Check sheet for the modelled part. Datum: model origin and axes. Units: mm. Face numbers are marked on the shaded views. A direction names the side the tool comes from. Round coordinates to 2 decimals unless told otherwise and drop trailing zeros. Order: outer loops, then holes, each group sorted by start corner. A loop starts at its lowest first (then second) coordinate and runs counter-clockwise, first axis right, second up.
```python
from build123d import *

# Parameters (mm, degrees)
F2_R    = 2.99999
F3_SIZE = 2


# Not quite as in the source:
# - a fillet or chamfer is up to 0.001 mm smaller than in the source, because OpenCascade refuses the exact size


with BuildPart() as f1:
    # F0 (on Top) → F1 (revolve)
    with BuildSketch(Plane.XY):
        Polygon((-62.0045285772, 2), (-62.0045285772, -10), (45.9954714228, -10), (45.9954714228, -5), (36.4192584626, 0), (31.4192584626, 0), (31.4192584626, -3), (26.4192584626, -3), (26.4192584626, 0), (21.4192584626, 0), (21.4192584626, 8), (11.4192584626, 8), (11.4192584626, 11), (1.4192584626, 11), (1.4192584626, 8), (-18.5807415374, 8), (-18.5807415374, 2), align=None)
    revolve(axis=Axis((-8.0045285772, -10, 0), (1, 0, 0)))

    # F2 (radius 3 in the source; OpenCascade refuses exactly that, so slightly less here)
    f2_edges = [f1.edges().sort_by_distance(p)[0] for p in [
        (-18.580742, -28, 0),
        (-18.580742, -22, 0),
    ]]
    fillet(f2_edges, radius=F2_R)

    # F3
    f3_edges = [f1.edges().sort_by_distance(p)[0] for p in [
        (21.419258, -28, 0),
        (-62.004529, -22, 0),
    ]]
    chamfer(f3_edges, length=F3_SIZE)


solid = f1.part
```
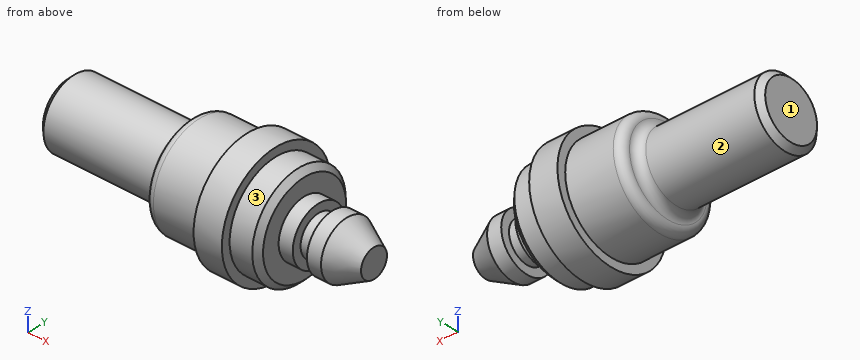
Item 1: Sectioned sample at A-A (x = -24). Record the cut outline in (y, z), and give its area (3 significant figures).
Answer:
outline: circle Ø24 at (-10, 0)
area: 452 mm2
Item 2: Sectioned sample at B-B (x = 32.5). Record the cut outline in (y, z).
Answer:
outline: circle Ø20 at (-10, 0)
Item 3: Scan lines: line 1 along X through (y, z) = (-10, -18.5); line 2 along Z through (x, y) = (10, -2); line 3 along X through (y, z) = (-7.5, -10). Record each from-to range of solid material in increasing order.
Answer:
line 1: x = 1.42 to 11.42
line 2: z = -19.42 to 19.42
line 3: x = -61.7 to 21.42
Item 4: Go/stop test with flat-tipped pins: P1, Ø1, axis at x = 23.5, z = 13.5, coming from the -Y side; P2, Ø12, axis at x = -4, z = -6.5, coming from the +Y side; P3, Ø5, axis at x = -32.5, y = -7, coming from the -Z side; P4, Ø2, axis at y = -24, z = -6.5, coming from the +X side. Record where each tip stops, or that it passes through.
Answer:
P1: passes through
P2: stops at y = 10.63
P3: stops at z = -11.99
P4: stops at x = 21.42
Item 5: Access from +Z, -Z, +X, -X, +Y, -Y to the whole of each face (thin tool, end or side, straight path). Record for the marked faces 1, 2 and 3.
Answer:
face 1: +Z, -Z, -X, +Y, -Y
face 2: -X
face 3: +X
